Input: part model. Units: mm. Frame: model coordinates. Round coordinates to 2 decimals unless told otherwise and drop trailing zeros. Order: outer loops, then holes, each group sorted by start corner. A loop starts at its lowest first (then second) coordinate and runs counter-clockwise, first axis right, second up.
Item 1: Cut plane C-C on z = -66. Output: boundary loops of the cut face in (x, y), then the cut area to 3 significant figures.
Item 2: Cut plane A-A on z = 0. Output: boundary loops of the cut face in (x, y).
Item 3: Line query: L1, parallel to X at y = 10, z = 0; L2, parallel to X at y = 2.6, z = 0; L3, parallel to Y at x = 203.5, z = 57. Output: solid intervals per line, ascending.
Item 4: Cut plane B-B on x = 136. Output: boundary loops of the cut face in (y, z).
Item 5: First-contact query: pin 1 (2 mm diameter, centred on x = -49.5, z = -54, fed in from +Y). Flat tip, straight axial feed; report the tip coordinate or a pass-through.
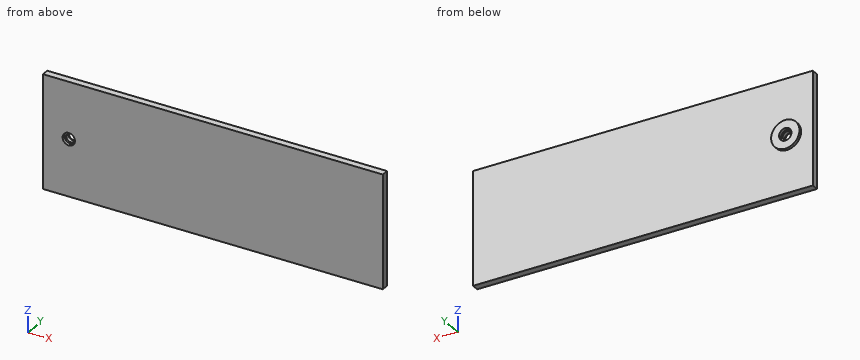
```python
from build123d import *

# Parameters (mm, degrees)
SKETCH1_W           = 609.6
SKETCH1_H           = 203.2
BOSS_EXTRUDE1_DEPTH = 12.7
SKETCH2_R           = 25.4
BOSS_EXTRUDE3_DEPTH = 5.08
SKETCH9_R           = 11.1125
CUT_EXTRUDE4_DEPTH  = 5.55625
CUT_EXTRUDE5_START  = -5.55625
SKETCH10_R          = 11.1125
CUT_EXTRUDE5_DEPTH  = 5.55625
SKETCH11_R          = 7.9375
CUT_EXTRUDE6_DEPTH  = 322.519859517


with BuildPart() as part:
    # Sketch1 → Boss-Extrude1 (new body)
    with BuildSketch(Plane(origin=(0, 0, 0), x_dir=(1, 0, 0), z_dir=(0, 1, 0))):
        Rectangle(SKETCH1_W, SKETCH1_H)
    extrude(amount=BOSS_EXTRUDE1_DEPTH)

    # Sketch2 → Boss-Extrude3 (add)
    with BuildSketch(Plane(origin=(0, 12.7, 0), x_dir=(1, 0, 0), z_dir=(0, 1, 0))):
        with Locations(Location((-258.510557857, 0, 0), (0, 0, 90))):
            Circle(SKETCH2_R)
    extrude(amount=BOSS_EXTRUDE3_DEPTH)

    # Sketch9 → Cut-Extrude4 (cut)
    with BuildSketch(Plane(origin=(0, 17.78, 0), x_dir=(1, 0, 0), z_dir=(0, 1, 0))):
        with Locations(Location((-258.510557857, 0, 0), (0, 0, 270))):
            Circle(SKETCH9_R)
    extrude(amount=-CUT_EXTRUDE4_DEPTH, mode=Mode.SUBTRACT)

    # Sketch10 → Cut-Extrude5 (cut)
    with BuildSketch(Plane(origin=(0, 0, 0), x_dir=(-1, 0, 0), z_dir=(0, -1, 0)).offset(CUT_EXTRUDE5_START)):
        with Locations(Location((258.510557857, 0, 0), (0, 0, 270))):
            Circle(SKETCH10_R)
    extrude(amount=CUT_EXTRUDE5_DEPTH, mode=Mode.SUBTRACT)

    # Sketch11 → Cut-Extrude6 (cut, through all)
    with BuildSketch(Plane(origin=(0, 12.22375, 0), x_dir=(1, 0, 0), z_dir=(0, 1, 0))):
        with Locations(Location((-258.510557857, 0, 0), (0, 0, 270))):
            Circle(SKETCH11_R)
    extrude(amount=-CUT_EXTRUDE6_DEPTH, mode=Mode.SUBTRACT)


solid = part.part
```
From the geometry:
1. outline: (-304.8, 0) - (304.8, 0) - (304.8, 12.7) - (-304.8, 12.7) - close
1. area: 7,740 mm2
2. outline: (-304.8, 0) - (-269.62, 0) - (-269.62, 5.56) - (-266.45, 5.56) - (-266.45, 12.22) - (-269.62, 12.22) - (-269.62, 17.78) - (-283.91, 17.78) - (-283.91, 12.7) - (-304.8, 12.7) - close; (-250.57, 5.56) - (-247.4, 5.56) - (-247.4, 0) - (304.8, 0) - (304.8, 12.7) - (-233.11, 12.7) - (-233.11, 17.78) - (-247.4, 17.78) - (-247.4, 12.22) - (-250.57, 12.22) - close
3. L1: x = -304.8 to -266.45, -250.57 to 304.8
3. L2: x = -304.8 to -269.62, -247.4 to 304.8
3. L3: y = 0 to 12.7
4. outline: (0, -101.6) - (12.7, -101.6) - (12.7, 101.6) - (0, 101.6) - close
5. pin 1: stops at y = 12.7
